CAD build for the part. Positions are in the model's coordinates, mm. A direction names the side the tool comes from. Round coordinates to 2 decimals unless told otherwise and drop trailing zeros. Loops run counter-clockwise (first coordinate to the right, second up) from the corner with the lowest first, then second, coordinate; pieces in that order, holes last.
from build123d import *

# Parameters (mm, degrees)
SKETCH_1_W                  = 21
SKETCH_1_H                  = 112
CUT_EXTRUDE_1_REACH         = 117.871
SKETCH_3_W                  = 42
SKETCH_3_H                  = 25
SKETCH_4_W                  = 15
SKETCH_4_H                  = 8
EXTRUDE_1_DEPTH             = 15
EXTRUDE_1_DIRECTION_2_REACH = 123.445
CUT_EXTRUDE_2_DEPTH         = 8
SKETCH_6_R                  = 2.6
CUT_EXTRUDE_3_DEPTH         = 8
SKETCH_7_R                  = 5.1
CUT_EXTRUDE_4_DEPTH         = 5
PATTERN_LINEAR_1_COUNT      = 2
PATTERN_LINEAR_1_PITCH      = 50
MIRROR_1_COPY_1_SKETCH_W    = 15
MIRROR_1_COPY_1_SKETCH_H    = 8
MIRROR_1_COPY_1_DEPTH       = 15
MIRROR_1_COPY_2_REACH       = 123.445
MIRROR_1_COPY_2_SKETCH_W    = 15
MIRROR_1_COPY_2_SKETCH_H    = 8
MIRROR_1_COPY_3_DEPTH       = 8
MIRROR_1_COPY_4_SKETCH_R    = 2.6
MIRROR_1_COPY_4_DEPTH       = 8
MIRROR_1_COPY_5_SKETCH_R    = 5.1
MIRROR_1_COPY_5_DEPTH       = 5
PATTERN_CIRCULAR_1_COUNT    = 2
PATTERN_CIRCULAR_1_ANGLE    = 90
CUT_EXTRUDE_6_REACH         = 121.503
CUT_EXTRUDE_6_END_RADIUS    = 21
SKETCH_9_W                  = 10
SKETCH_9_H                  = 12


with BuildPart() as part:
    # Эскиз1 → Повернуть1 (revolve)
    with BuildSketch(Plane(origin=(0, 0, 0), x_dir=(1, 0, 0), z_dir=(0, 1, 0))):
        with Locations((10.5, 56)):
            Rectangle(SKETCH_1_W, SKETCH_1_H)
    revolve(axis=Axis((0, 0, 0), (0, 0, -1)))

    # Эскиз2 → Вырез-Повернуть1 (revolve, cut)
    with BuildSketch(Plane(origin=(0, 0, 0), x_dir=(1, 0, 0), z_dir=(0, 1, 0)), mode=Mode.PRIVATE) as cut_revolve_1_sk:
        Polygon((0, 0), (12.5, 0), (12.5, 9.8), (11, 9.8), (11, 98.5), (5, 98.5), (5, 107.5), (11, 107.5), (11, 112), (0, 112), align=None)
    revolve(cut_revolve_1_sk.sketch.rotate(Axis((0, 0, -112), (0, 0, 1)), 180), axis=Axis((0, 0, -112), (0, 0, 1)), mode=Mode.SUBTRACT)

    # Вырез-Вытянуть1: up to this face of the body (flat: up to its plane)
    cut_extrude_1_end = Plane(part.part.faces().sort_by_distance((-20.406030304, 0, -112))[0])
    # Эскиз3 → Вырез-Вытянуть1 (cut, up to the picked face)
    with BuildSketch(Plane.XY, mode=Mode.PRIVATE) as cut_extrude_1_sk1:
        with Locations((0, -12.5)):
            Rectangle(SKETCH_3_W, SKETCH_3_H)
    cut_extrude_1_tool1 = split(extrude(cut_extrude_1_sk1.sketch, amount=-CUT_EXTRUDE_1_REACH, mode=Mode.PRIVATE), bisect_by=cut_extrude_1_end, keep=Keep.BOTH, mode=Mode.PRIVATE)
    add(cut_extrude_1_tool1.solids().sort_by(Axis((0, -12.5, 0), (0, 0, -1)))[0], mode=Mode.SUBTRACT)

    # Эскиз4 → Бобышка-Вытянуть1 (add)
    with BuildSketch(Plane(origin=(21, 0, 0), x_dir=(0, 0, -1), z_dir=(1, 0, 0))):
        with Locations((31, 4)):
            Rectangle(SKETCH_4_W, SKETCH_4_H)
    extrude_1 = extrude(amount=EXTRUDE_1_DEPTH)

    # Эскиз4 → Бобышка-Вытянуть1 direction 2 (add, up to next)
    with BuildSketch(Plane(origin=(21, 0, 0), x_dir=(0, 0, -1), z_dir=(1, 0, 0)), mode=Mode.PRIVATE) as extrude_1_direction_2_sk1:
        with Locations((31, 4)):
            Rectangle(SKETCH_4_W, SKETCH_4_H)
    extrude_1_direction_2_tool1 = extrude(extrude_1_direction_2_sk1.sketch, amount=-EXTRUDE_1_DIRECTION_2_REACH, mode=Mode.PRIVATE) - part.part
    extrude_1_direction_2 = extrude_1_direction_2_tool1.solids().sort_by_distance((21, 4, -31))[0]
    add(extrude_1_direction_2)

    # Эскиз5 → Вырез-Вытянуть2 (cut)
    with BuildSketch(Plane(origin=(0, 8, 0), x_dir=(1, 0, 0), z_dir=(0, 1, 0))):
        with BuildLine():
            Line((28.5, 38.5), (43.5, 38.5))
            Line((43.5, 38.5), (43.5, 23.5))
            Line((43.5, 23.5), (28.5, 23.5))
            ThreePointArc((28.5, 23.5), (36, 31), (28.5, 38.5))
        make_face()
    cut_extrude_2 = extrude(amount=-CUT_EXTRUDE_2_DEPTH, mode=Mode.SUBTRACT)

    # Эскиз6 → Вырез-Вытянуть3 (cut)
    with BuildSketch(Plane(origin=(0, 8, 0), x_dir=(1, 0, 0), z_dir=(0, 1, 0))):
        with Locations(Location((28.5, 31, 0), (0, 0, 270))):
            Circle(SKETCH_6_R)
    cut_extrude_3 = extrude(amount=-CUT_EXTRUDE_3_DEPTH, mode=Mode.SUBTRACT)

    # Эскиз7 → Вырез-Вытянуть4 (cut)
    with BuildSketch(Plane(origin=(0, 8, 0), x_dir=(1, 0, 0), z_dir=(0, 1, 0))):
        with Locations(Location((28.5, 31, 0), (0, 0, 270))):
            Circle(SKETCH_7_R)
    cut_extrude_4 = extrude(amount=-CUT_EXTRUDE_4_DEPTH, mode=Mode.SUBTRACT)

    # Линейный массив1: Бобышка-Вытянуть1, Бобышка-Вытянуть1 direction 2, Вырез-Вытянуть2, Вырез-Вытянуть3, Вырез-Вытянуть4 ×2
    with Locations(*[(0, 0, -i * PATTERN_LINEAR_1_PITCH) for i in range(1, PATTERN_LINEAR_1_COUNT)]):
        add(extrude_1)
        add(extrude_1_direction_2)
        add(cut_extrude_2, mode=Mode.SUBTRACT)
        add(cut_extrude_3, mode=Mode.SUBTRACT)
        add(cut_extrude_4, mode=Mode.SUBTRACT)

    # Зеркальное отражение1: Бобышка-Вытянуть1, Бобышка-Вытянуть1 direction 2, Вырез-Вытянуть2, Вырез-Вытянуть3, Вырез-Вытянуть4 across plane
    add(extrude_1.mirror(Plane(origin=(0, 0, 0), x_dir=(0, 0, 1), z_dir=(1, 0, 0))))
    add(extrude_1_direction_2.mirror(Plane(origin=(0, 0, 0), x_dir=(0, 0, 1), z_dir=(1, 0, 0))))
    add(cut_extrude_2.mirror(Plane(origin=(0, 0, 0), x_dir=(0, 0, 1), z_dir=(1, 0, 0))), mode=Mode.SUBTRACT)
    add(cut_extrude_3.mirror(Plane(origin=(0, 0, 0), x_dir=(0, 0, 1), z_dir=(1, 0, 0))), mode=Mode.SUBTRACT)
    add(cut_extrude_4.mirror(Plane(origin=(0, 0, 0), x_dir=(0, 0, 1), z_dir=(1, 0, 0))), mode=Mode.SUBTRACT)

    # Зеркальное отражение1 copy 1 sketch → Зеркальное отражение1 copy 1 (add)
    with BuildSketch(Plane(origin=(-21, 0, -50), x_dir=(0, 0, -1), z_dir=(-1, 0, 0))):
        with Locations((31, -4)):
            Rectangle(MIRROR_1_COPY_1_SKETCH_W, MIRROR_1_COPY_1_SKETCH_H)
    extrude(amount=MIRROR_1_COPY_1_DEPTH)

    # Зеркальное отражение1 copy 2 sketch → Зеркальное отражение1 copy 2 (add, up to next)
    with BuildSketch(Plane(origin=(-21, 0, -50), x_dir=(0, 0, -1), z_dir=(-1, 0, 0)), mode=Mode.PRIVATE) as mirror_1_copy_2_sk1:
        with Locations((31, -4)):
            Rectangle(MIRROR_1_COPY_2_SKETCH_W, MIRROR_1_COPY_2_SKETCH_H)
    mirror_1_copy_2_tool1 = extrude(mirror_1_copy_2_sk1.sketch, amount=-MIRROR_1_COPY_2_REACH, mode=Mode.PRIVATE) - part.part
    add(mirror_1_copy_2_tool1.solids().sort_by_distance((-21, 4, -81))[0])

    # Зеркальное отражение1 copy 3 sketch → Зеркальное отражение1 copy 3 (cut)
    with BuildSketch(Plane(origin=(0, 8, -50), x_dir=(-1, 0, 0), z_dir=(0, 1, 0))):
        with BuildLine():
            Line((28.5, -38.5), (43.5, -38.5))
            Line((43.5, -38.5), (43.5, -23.5))
            Line((43.5, -23.5), (28.5, -23.5))
            ThreePointArc((28.5, -23.5), (36, -31), (28.5, -38.5))
        make_face()
    extrude(amount=-MIRROR_1_COPY_3_DEPTH, mode=Mode.SUBTRACT)

    # Зеркальное отражение1 copy 4 sketch → Зеркальное отражение1 copy 4 (cut)
    with BuildSketch(Plane(origin=(0, 8, -50), x_dir=(-1, 0, 0), z_dir=(0, 1, 0))):
        with Locations((28.5, -31)):
            Circle(MIRROR_1_COPY_4_SKETCH_R)
    extrude(amount=-MIRROR_1_COPY_4_DEPTH, mode=Mode.SUBTRACT)

    # Зеркальное отражение1 copy 5 sketch → Зеркальное отражение1 copy 5 (cut)
    with BuildSketch(Plane(origin=(0, 8, -50), x_dir=(-1, 0, 0), z_dir=(0, 1, 0))):
        with Locations((28.5, -31)):
            Circle(MIRROR_1_COPY_5_SKETCH_R)
    extrude(amount=-MIRROR_1_COPY_5_DEPTH, mode=Mode.SUBTRACT)

    # Эскиз8 → Сверление под метчик M51 (revolve, cut)
    with BuildSketch(Plane(origin=(11.313708499, 11.313708499, 0), x_dir=(0, -1, 0), z_dir=(1, 0, 0))):
        Polygon((0, 0), (0, 26.2618073), (2.1, 25), (2.1, 0), align=None)
    hole_wizard_m51 = revolve(axis=Axis((11.313708499, 11.313708499, 6.35), (0, 0, -1)), mode=Mode.SUBTRACT)

    # Круговой массив1: Сверление под метчик M51 ×2 about axis
    pattern_circular_1_axis = Axis((0, 0, 0), (0, 0, 1))
    for i in range(1, PATTERN_CIRCULAR_1_COUNT):
        add(hole_wizard_m51.rotate(pattern_circular_1_axis, i * PATTERN_CIRCULAR_1_ANGLE / (PATTERN_CIRCULAR_1_COUNT - 1)), mode=Mode.SUBTRACT)

    # Зеркальное отражение2: Сверление под метчик M51 across plane
    add(hole_wizard_m51.mirror(Plane.XY.offset(-56)), mode=Mode.SUBTRACT)

    # Зеркальное отражение2 copy 1 sketch → Зеркальное отражение2 copy 1 (revolve, cut)
    with BuildSketch(Plane(origin=(-11.313708499, 11.313708499, -112), x_dir=(1, 0, 0), z_dir=(0, 1, 0))):
        Polygon((0, 0), (0, -26.2618073), (2.1, -25), (2.1, 0), align=None)
    revolve(axis=Axis((-11.313708499, 11.313708499, -118.35), (0, 0, -1)), mode=Mode.SUBTRACT)

    # Вырез-Вытянуть6: up to this cylinder (the profile starts inside it)
    cut_extrude_6_end = Plane(origin=(0, 0, -101.5), z_dir=(0, 0, 1)) * Cylinder(CUT_EXTRUDE_6_END_RADIUS, 286.006, mode=Mode.PRIVATE)
    # Эскиз9 → Вырез-Вытянуть6 (cut, up to the surface)
    with BuildSketch(Plane(origin=(0, 0, 0), x_dir=(1, 0, 0), z_dir=(0, 1, 0)), mode=Mode.PRIVATE) as cut_extrude_6_sk1:
        with Locations((0, 101.5)):
            Rectangle(SKETCH_9_W, SKETCH_9_H)
    cut_extrude_6_tool1 = extrude(cut_extrude_6_sk1.sketch, amount=CUT_EXTRUDE_6_REACH, mode=Mode.PRIVATE) & cut_extrude_6_end
    add(cut_extrude_6_tool1.solids().sort_by_distance((0, 0, -101.5))[0], mode=Mode.SUBTRACT)


solid = part.part
Item 1: Cut at A-A (z = -81). List the corners of the cut face in (x, y).
Verdict:
outline: (-36, 0) - (-31.1, 0) - (-31.1, 3) - (-33.6, 3) - (-33.6, 8) - (-36, 8) - close; (-25.9, 0) - (-11, 0) arc R11 cw to (11, 0) - (25.9, 0) - (25.9, 3) - (23.4, 3) - (23.4, 8) - (19.42, 8) arc R21 ccw to (-19.42, 8) - (-23.4, 8) - (-23.4, 3) - (-25.9, 3) - close; (31.1, 0) - (36, 0) - (36, 8) - (33.6, 8) - (33.6, 3) - (31.1, 3) - close
Item 2: Cut at B-B (x = 0). List the corners of the cut face in (y, z), plus the area to 3 significant figures.
Verdict:
outline: (11, -112) - (21, -112) - (21, -107.5) - (11, -107.5) - close; (11, -95.5) - (21, -95.5) - (21, 0) - (12.5, 0) - (12.5, -9.8) - (11, -9.8) - close
area: 985 mm2
Item 3: Mould opens along X. For faces 1 (the flat face through (-26, 3, -29)), 2 (the cylindrical face through (-36, 4, -81)), 3 (the flat face through (-24, 4, -23.5)) say: released by +X, released by -X, zero draft, split by the parting line, or undercut.
Verdict:
face 1: undercut
face 2: released by -X
face 3: zero draft
Item 4: Cut at C-C (y = 6.5). State how many separate pieces and enclosed holes the cut face has, plus the area to 3 significant figures.
Verdict:
separate pieces: 2
enclosed holes: 4
area: 3,060 mm2
Item 5: Wall check: L1, parallel to Z at x = -28.5, y = 1.85; L2, parallel to Z at x = -28.5, y = 5.5; L3, parallel to Z at x = 23, y = 6. Give the ranges that are in metal, low to high.
Verdict:
L1: z = -88.5 to -83.6, -78.4 to -73.5, -38.5 to -33.6, -28.4 to -23.5
L2: z = -88.5 to -86.1, -75.9 to -73.5, -38.5 to -36.1, -25.9 to -23.5
L3: z = -88.5 to -73.5, -38.5 to -23.5
Item 6: Flat gauge pins, fed straight in: P1, Ø3, axis at x = 27.5, z = -28.5, coming from the +Y side; P2, Ø1.8, axis at x = 7, y = 5.5, coming from the -Z side; P3, Ø12, axis at x = 28, z = -29, coming from the +Y side; P4, Ø3, axis at x = -28.5, z = -31, coming from the -Y side. Where does each tip first touch, or does it go through?
Verdict:
P1: stops at y = 3
P2: stops at z = -107.5
P3: stops at y = 8
P4: passes through
Item 7: 3-axis set-ups, long thin cutter, end or side, ignore diameter. For faces 4 (the flat face through (-7, 4, -107.5)), 5 (the cylindrical face through (-27.836, 5.535, -75.943)), 6 (the flat face through (0, 15, -107.5)), 7 (the flat face through (24, 8, -78)): which of +Z, -Z, +X, -X, +Y, -Y reach the whole face in a straight line?
Verdict:
face 4: -Z, -Y
face 5: +Y
face 6: +Y, -Y
face 7: +Z, -Z, +X, +Y
Item 8: Cut at D-D (x = 7.5). List the corners of the cut face in (y, z).
Verdict:
outline: (0, -107.5) - (8.05, -107.5) - (8.05, -112) - (19.62, -112) - (19.62, 0) - (10, 0) - (10, -9.8) - (8.05, -9.8) - (8.05, -98.5) - (0, -98.5) - close
